Autodesk Inventor part; units mm, degrees
ref_plane "YZ Plane" through (0, 0, 0) normal (1, 0, 0) x (0, 1, 0)
ref_plane "XZ Plane" through (0, 0, 0) normal (0, 1, 0) x (-1, 0, 0)
ref_plane "XY Plane" through (0, 0, 0) normal (0, 0, 1) x (1, 0, 0)
sketch "Block1" plane through (0, 0, 0) normal (0, 0, 1) x (1, 0, 0)
  circle A0 centre (74.029, 24.2723) radius 1
  line L0 (49.279, 30.4723) -> (71.779, 30.4723)
  line L1 (71.779, 30.4723) -> (71.779, 18.0723)
  line L2 (71.779, 18.0723) -> (49.279, 18.0723)
  line L3 (49.279, 18.0723) -> (49.279, 30.4723)
  line L4 (49.279, 30.4723) -> (44.779, 30.4723)
  line L5 (44.779, 30.4723) -> (44.779, 18.0723)
  line L6 (44.779, 18.0723) -> (49.279, 18.0723)
  line L7 (49.279, 18.0723) -> (49.279, 30.4723)
  line L8 (71.779, 30.4723) -> (76.279, 30.4723)
  line L9 (76.279, 30.4723) -> (76.279, 18.0723)
  line L10 (76.279, 18.0723) -> (71.779, 18.0723)
  line L11 (71.779, 18.0723) -> (71.779, 30.4723)
  line L12 (44.779, 24.2723) -> (76.279, 24.2723) construction
  line L13 (47.029, 30.4723) -> (47.029, 18.0723) construction
  circle A1 centre (47.029, 24.2723) radius 1
  line L14 (74.029, 30.4723) -> (74.029, 18.0723) construction
  point P0 (60.979, 24.0984)
  dimension "d7" = 22.5
  dimension "d8" = 12.4
  dimension "d9" = 4.5
  dimension "d10" = 4.5
  dimension "d11" = 2
  dimension "d12" = 2
sketch "Sketch1" plane through (0, 0, 0) normal (0, 0, 1) x (1, 0, 0)
  line L0 (-92.7646, -8.503) -> (-89.7646, -8.503)
  line L1 (-89.7646, -8.503) -> (-89.7646, -11.753)
  line L2 (-89.7646, -11.753) -> (-92.7646, -11.753)
  line L3 (-92.7646, -11.753) -> (-92.7646, -8.503)
  line L4 (-92.7646, -21.6527) -> (-89.7646, -21.6527)
  line L5 (-89.7646, -21.6527) -> (-89.7646, -21.7527)
  line L6 (-89.7646, -21.7527) -> (-92.7646, -21.7527)
  line L7 (-92.7646, -21.7527) -> (-92.7646, -21.6527)
  line L8 (-51.3097, 52.8088) -> (28.6903, 52.8088)
  line L9 (28.6903, 52.8088) -> (28.6903, 26.8088)
  line L10 (28.6903, 26.8088) -> (-51.3097, 26.8088)
  line L11 (-51.3097, 26.8088) -> (-51.3097, 52.8088)
  line L12 (-51.3097, 39.8088) -> (28.6903, 39.8088) construction
  line L13 (-21.3097, 46.8088) -> (-18.0597, 46.8088)
  line L14 (-18.0597, 46.8088) -> (-18.0597, 32.8088)
  line L15 (-18.0597, 32.8088) -> (-21.3097, 32.8088)
  line L16 (-21.3097, 32.8088) -> (-21.3097, 46.8088)
  line L17 (-21.3097, 39.8088) -> (-18.0597, 39.8088) construction
  line L18 (-38.3097, 52.8088) -> (-38.3097, 26.8088) construction
  arc A0 (-38.3097, 52.8088) -> (-38.3097, 26.8088) centre (-38.3097, 39.8088) ccw
  line L19 (-11.3097, 52.8088) -> (-11.3097, 26.8088) construction
  line L20 (15.6903, 52.8088) -> (15.6903, 26.8088) construction
  arc A1 (15.6903, 26.8088) -> (15.6903, 52.8088) centre (15.6903, 39.8088) ccw
  circle A2 centre (-5.5597, 39.8088) radius 1
  line L21 (19.1903, 33.6088) -> (-3.3097, 33.6088)
  line L22 (-3.3097, 33.6088) -> (-3.3097, 46.0088)
  line L23 (-3.3097, 46.0088) -> (19.1903, 46.0088)
  line L24 (19.1903, 46.0088) -> (19.1903, 33.6088)
  line L25 (19.1903, 33.6088) -> (23.6903, 33.6088)
  line L26 (23.6903, 33.6088) -> (23.6903, 46.0088)
  line L27 (23.6903, 46.0088) -> (19.1903, 46.0088)
  line L28 (19.1903, 46.0088) -> (19.1903, 33.6088)
  line L29 (-3.3097, 33.6088) -> (-7.8097, 33.6088)
  line L30 (-7.8097, 33.6088) -> (-7.8097, 46.0088)
  line L31 (-7.8097, 46.0088) -> (-3.3097, 46.0088)
  line L32 (-3.3097, 46.0088) -> (-3.3097, 33.6088)
  line L33 (23.6903, 39.8088) -> (-7.8097, 39.8088) construction
  line L34 (21.4403, 33.6088) -> (21.4403, 46.0088) construction
  circle A3 centre (21.4403, 39.8088) radius 1
  line L35 (-5.5597, 33.6088) -> (-5.5597, 46.0088) construction
  point P0 (0, 0)
  dimension "d0" = 3
  dimension "mat" = 3.25
  dimension "d2" = 3
  dimension "d3" = 0.1
  dimension "d23" = 80
  dimension "d24" = 26
  dimension "d25" = 5
  dimension "d29" = 3.25
  dimension "d30" = 14
  dimension "d31" = 30
  dimension "d38" = 13
  dimension "d39" = 13
extrude "Extrusion5" add sketch "Sketch1" along normal blind 3.25 contours L8 A1 L10 A0 | L24 L27 L26 L25 | L29 L30 L31 L22
equation "\"d29\" = mat"
equation "\"d40\" = mat"
properties part number "arm-servo"
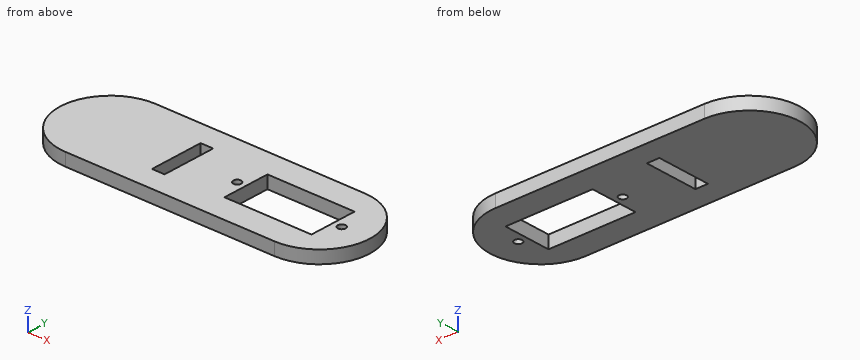
Could you check a few things on this model? Use its own coordinates, in mm. Give positions to 0.01 mm unless a question says otherwise; leave off trailing zeros. Order: outer loops, then holes, each group sorted by start corner. A loop starts at its lowest first (then second) coordinate and runs counter-clockwise, first axis right, second up. Notation, with made-up numbers: (72, 28.25) - (76, 28.25) arc R18 cw to (76, 39.25) - close; hole circle Ø9 at (52.5, 75.25). An arc over 180 degrees is marked (long way). One line per question, with ' | ' between items. Start each with the question number.
Item 1: I want a section at A-A on x = 3.5. Write out the boundary of the cut face in (y, z), then the cut area to 3 significant figures.
Item 2: I need wall thicknesses on probe 1 along X at (y, z) = (39.75, 0.9); probe 2 along Y at (x, z) = (-1.5, 2.4); probe 3 along X at (y, z) = (41.75, 0.4). Which ranges of each line are inside material? Lowest first, please. Write a range as [from, to].
Item 3: I'm going to push a flat-ended pin straight in: pin 1 Ø1.6 at (y, z) = (42, 2) entering from -X. Where does the tip first touch, or does it pass through?
Item 4: I want a section at D-D on y = 44.5. Write out the boundary of the cut face in (x, z).
Item 5: I want a section at C-C on z = 0.8. Write out the boundary of the cut face in (x, y), then the cut area to 3 significant figures.
Item 6: I want a section at B-B on y = 36.25. Write out the boundary of the cut face in (x, z).
Verdict:
1) outline: (26.81, 0) - (33.61, 0) - (33.61, 3.25) - (26.81, 3.25) - close; (46.01, 0) - (52.81, 0) - (52.81, 3.25) - (46.01, 3.25) - close | area: 44.2 mm^2
2) probe 1: [-51.31, -21.31], [-18.06, -6.56], [-4.56, -3.31], [19.19, 20.44], [22.44, 28.69] | probe 2: [26.81, 33.61], [46.01, 52.81] | probe 3: [-51.16, -21.31], [-18.06, -3.31], [19.19, 28.54]
3) pin 1: x = -51.24
4) outline: (-50.43, 0) - (-21.31, 0) - (-21.31, 3.25) - (-50.43, 3.25) - close; (-18.06, 0) - (-3.31, 0) - (-3.31, 3.25) - (-18.06, 3.25) - close; (19.19, 0) - (27.81, 0) - (27.81, 3.25) - (19.19, 3.25) - close
5) outline: (-38.31, 26.81) - (15.69, 26.81) arc R13 ccw to (15.69, 52.81) - (-38.31, 52.81) arc R13 ccw to start; hole (-21.31, 32.81) - (-18.06, 32.81) - (-18.06, 46.81) - (-21.31, 46.81) - close; hole circle Ø2 at (-5.56, 39.81); hole (-3.31, 33.61) - (19.19, 33.61) - (19.19, 46.01) - (-3.31, 46.01) - close; hole circle Ø2 at (21.44, 39.81) | area: 1,600 mm^2
6) outline: (-50.81, 0) - (-21.31, 0) - (-21.31, 3.25) - (-50.81, 3.25) - close; (-18.06, 0) - (-3.31, 0) - (-3.31, 3.25) - (-18.06, 3.25) - close; (19.19, 0) - (28.19, 0) - (28.19, 3.25) - (19.19, 3.25) - close
